from build123d import *

# Parameters (mm, degrees)
BOSS_EXTRUDE1_DEPTH = 67
BOSS_EXTRUDE2_START = 13
SKETCH1_3_R         = 4
BOSS_EXTRUDE2_DEPTH = 13
BOSS_EXTRUDE3_START = -67
SKETCH1_4_R         = 6
BOSS_EXTRUDE3_DEPTH = 3
CUT_EXTRUDE1_DEPTH  = 11
SKETCH3_R           = 1.5
CUT_EXTRUDE2_DEPTH  = 4


with BuildPart() as part:
    # Sketch1 → Boss-Extrude1 (new body)
    with BuildSketch(Plane(origin=(0, 0, 0), x_dir=(1, 0, 0), z_dir=(0, 1, 0))):
        with BuildLine():
            Line((1.5, 1.5), (1.5, 3.708099244))
            ThreePointArc((1.5, 3.708099244), (0, 4), (-1.5, 3.708099244))
            Line((-1.5, 3.708099244), (-1.5, 1.5))
            Line((-1.5, 1.5), (-3.708099244, 1.5))
            ThreePointArc((-3.708099244, 1.5), (-4, 0), (-3.708099244, -1.5))
            Line((-3.708099244, -1.5), (-1.5, -1.5))
            Line((-1.5, -1.5), (-1.5, -3.708099244))
            ThreePointArc((-1.5, -3.708099244), (0, -4), (1.5, -3.708099244))
            Line((1.5, -3.708099244), (1.5, -1.5))
            Line((1.5, -1.5), (3.708099244, -1.5))
            ThreePointArc((3.708099244, -1.5), (3.92634671, -0.76406905), (4, 0))
            ThreePointArc((4, 0), (3.92634671, 0.76406905), (3.708099244, 1.5))
            Line((3.708099244, 1.5), (1.5, 1.5))
        make_face()
    extrude(amount=-BOSS_EXTRUDE1_DEPTH)

    # Sketch1_3 → Boss-Extrude2 (add)
    with BuildSketch(Plane(origin=(0, 0, 0), x_dir=(1, 0, 0), z_dir=(0, 1, 0)).offset(BOSS_EXTRUDE2_START)):
        with Locations(Location((0, 0, 0), (0, 0, 270))):
            Circle(SKETCH1_3_R)
    extrude(amount=-BOSS_EXTRUDE2_DEPTH)

    # Sketch1_4 → Boss-Extrude3 (add)
    with BuildSketch(Plane(origin=(0, 0, 0), x_dir=(1, 0, 0), z_dir=(0, 1, 0)).offset(BOSS_EXTRUDE3_START)):
        with Locations(Location((0, 0, 0), (0, 0, 270))):
            Circle(SKETCH1_4_R)
    extrude(amount=-BOSS_EXTRUDE3_DEPTH)

    # Sketch2 → Cut-Extrude1 (cut)
    with BuildSketch(Plane(origin=(0, 13, 0), x_dir=(1, 0, 0), z_dir=(0, 1, 0))):
        with BuildLine():
            Line((3.708099244, 1.5), (3.708099244, -1.5))
            ThreePointArc((3.708099244, -1.5), (4, 0), (3.708099244, 1.5))
        make_face()
    cut_extrude1 = extrude(amount=-CUT_EXTRUDE1_DEPTH, mode=Mode.SUBTRACT)

    # Sketch3 → Cut-Extrude2 (cut)
    with BuildSketch(Plane(origin=(3.708099244, 0, 0), x_dir=(0, 0, -1), z_dir=(1, 0, 0))):
        with Locations((0, 8)):
            Circle(SKETCH3_R)
    cut_extrude2 = extrude(amount=-CUT_EXTRUDE2_DEPTH, mode=Mode.SUBTRACT)

    # Mirror1: Cut-Extrude1, Cut-Extrude2 across plane
    add(cut_extrude1.mirror(Plane(origin=(0, 0, 0), x_dir=(0, 0, 1), z_dir=(1, 0, 0))), mode=Mode.SUBTRACT)
    add(cut_extrude2.mirror(Plane(origin=(0, 0, 0), x_dir=(0, 0, 1), z_dir=(1, 0, 0))), mode=Mode.SUBTRACT)


solid = part.part
Geometry check sheet. Reference: the model listing, model coordinates, mm. A direction names the side the tool comes from. Give positions to 0.01 mm unless a question says otherwise; leave off trailing zeros. Loops run counter-clockwise (first coordinate to the right, second up) from the corner with the lowest first, then second, coordinate; pieces in that order, holes last.
(1) Section check A-A on y = -24. Record the cut outline in (x, z).
From the geometry:
outline: (-3.71, -1.5) - (-1.5, -1.5) - (-1.5, -3.71) arc R4 ccw to (1.5, -3.71) - (1.5, -1.5) - (3.71, -1.5) arc R4 ccw to (3.71, 1.5) - (1.5, 1.5) - (1.5, 3.71) arc R4 ccw to (-1.5, 3.71) - (-1.5, 1.5) - (-3.71, 1.5) arc R4 ccw to start
(2) Set-up check for faces 1 (the flat face through (3.708, 11, 0)), 2 (the flat face through (1.5, -33, -3)), 3 (the flat face through (-1.5, -33, 3)): record each of +Z, -Z, +X, -X, +Y, -Y from which the full face is reachable in a straight line by a thin tool's end or side.
From the geometry:
face 1: +Z, -Z, +X, +Y
face 2: -Z, +X
face 3: +Z, -X
(3) Release check for a two-part mould opening along Y. For faces 4 (the flat face through (0, -70, 0)), 5 (the flat face through (3.708, 4, 0)), 6 (the flat face through (-2, 0, -2)) record: released by +Y, released by -Y, zero draft, split by the parting line, or undercut.
From the geometry:
face 4: released by -Y
face 5: zero draft
face 6: undercut
(4) Section check C-C on z = 2.5. Record the cut outline in (x, y).
From the geometry:
outline: (-5.45, -70) - (5.45, -70) - (5.45, -67) - (1.5, -67) - (1.5, 0) - (3.12, 0) - (3.12, 13) - (-3.12, 13) - (-3.12, 0) - (-1.5, 0) - (-1.5, -67) - (-5.45, -67) - close
(5) Section check B-B on z = -2.25. Record the cut outline in (x, y).
From the geometry:
outline: (-5.56, -70) - (5.56, -70) - (5.56, -67) - (1.5, -67) - (1.5, 0) - (3.31, 0) - (3.31, 13) - (-3.31, 13) - (-3.31, 0) - (-1.5, 0) - (-1.5, -67) - (-5.56, -67) - close
(6) Thickness scan on L1, parallel to Y at x = -1.7, z = 0; L2, parallel to Y at x = 2.5, z = -2.5; L3, parallel to X at y = -8, z = 3.5. Record the ranges inside material, lowest first.
From the geometry:
L1: y = -70 to 6.5, 9.5 to 13
L2: y = -70 to -67, 0 to 13
L3: x = -1.5 to 1.5
(7) Depth check by flat-ended pin: pin 1 Ø1.8 at (x, y) = (2.5, -24.5) entering from +Z; pin 2 Ø2 at (y, z) = (-3.5, 3) entering from +X; pin 3 Ø4 at (y, z) = (8, 0) entering from +X. Enter the tip coordinate at first touch or a pass-through.
From the geometry:
pin 1: stops at z = 1.5
pin 2: stops at x = 1.5
pin 3: stops at x = 3.71
